Work out the finished part from the listing and answer in its coordinate system (mm). Coordinates: 2 decimals unless noted, no trailing zeros. Loops run counter-clockwise (first coordinate to the right, second up) from the corner with the lowest first, then second, coordinate; pieces in that order, holes last. Notation, with made-up numbers: (0.25, 73.25) -> (58.25, 73.25) arc R35 cw to (58.25, 111.25) -> close; hole circle Ø7 at (-31.5, 33). An arc over 180 degrees is marked (long way). Use a Markdown table: item, result.
from build123d import *

# Parameters (mm, degrees)
F1_DEPTH = 50.8
F2_R     = 49.05682
F3_R     = 49.0474


with BuildPart() as f1:
    # F0 (on Top) → F1 (new body)
    with BuildSketch(Plane.XY):
        Polygon((-49.864192, 53.976998), (-154.979095, 53.976998), (-154.979095, -239.501879), (-49.864192, -239.501879), (-49.864192, -202.062055), align=None)
    extrude(amount=F1_DEPTH)

    # F2
    f2_edges = [f1.edges().sort_by_distance(p)[0] for p in [
        (-102.421643, -239.501879, 50.8),
    ]]
    fillet(f2_edges, radius=F2_R)

    # F3
    f3_edges = [f1.edges().sort_by_distance(p)[0] for p in [
        (-102.421643, 53.976998, 50.8),
    ]]
    fillet(f3_edges, radius=F3_R)


solid = f1.part
Q1. Given pin 1 Ø12 at (x, z) = (-90.5, 12) entering from +Y; pin 2 Ø6 at (x, z) = (-126.5, 41.5) entering from +Y; pin 3 Ø4 at (x, z) = (-106.5, 43.5) entering from +Y, each flat-ended and moving along its own axis, determine where each tip first touches the part or whether it passes through.
Solved:
| item | result |
|---|---|
| pin 1 | y = 53.79 |
| pin 2 | y = 37.41 |
| pin 3 | y = 33.67 |
Q2. Section C-C on z = 43 is taken. Determine the outline of the cut face in (x, y).
Solved:
| item | result |
|---|---|
| outline | (-154.98, -216.99) -> (-49.86, -216.99) -> (-49.86, 31.47) -> (-154.98, 31.47) -> close |
Q3. Consider line 1 (Y direction, x = -105.5, z = 4); line 2 (Z direction, x = -142, y = 40); line 3 (Y direction, x = -97, z = 22). Determine where each line is inside the solid, lowest interval first. Write a range as [from, to].
Solved:
| item | result |
|---|---|
| line 1 | [-239.45, 53.93] |
| line 2 | [0, 36.04] |
| line 3 | [-235.12, 49.6] |
Q4. Section B-B on z = 24 is taken. Determine the outline of the cut face in (x, y), and give its area (3 significant figures).
Solved:
| item | result |
|---|---|
| outline | (-154.98, -234.16) -> (-49.86, -234.16) -> (-49.86, 48.64) -> (-154.98, 48.64) -> close |
| area | 29,700 mm² |
Q5. Section A-A on x = -137 is taken. Determine the outline of the cut face in (y, z), and give its area (3 significant figures).
Solved:
| item | result |
|---|---|
| outline | (-239.5, 0) -> (53.98, 0) -> (53.98, 1.75) arc R49.05 ccw to (4.93, 50.8) -> (-190.45, 50.8) arc R49.06 ccw to (-239.5, 1.74) -> close |
| area | 13,900 mm² |
